Could you check a few things on this model? Use its own coordinates, in mm. A direction names the side the tool comes from. Round coordinates to 2 decimals unless told otherwise and drop trailing zeros. Loops run counter-clockwise (first coordinate to the right, second up) from the corner with the lowest first, then second, coordinate; pieces in that order, holes last. Notation, with made-up numbers: (29.5, 65) -> (41.5, 65) arc R16 cw to (41.5, 69) -> close; hole circle Ø3 at (-5.75, 33). An arc over 180 degrees is marked (long way). Put each result on its own line as item: value. Start each with the question number.
1. Which directions (+Z, -Z, +X, -X, +Y, -Y) give clear straight access to the entire face, cutting with the end or side of a thin tool? Please do faces 4 (the flat face through (29.75, 2, 19)), 5 (the cylindrical face through (22.57, 1.77, 37.4)).
2. I'm going to push a flat-ended pin straight in: P1, Ø3, axis at x = 34, z = 34, coming from the +Y side. Where does the tip first touch, or does it pass through?
3. Imagine slicing it at D-D, the plane x = 25.5. Please give me the cut outline in (y, z), and give its area (3 significant figures).
4. Imagine slicing it at A-A, the plane z = 34. Count the separate pieces of the cut face and the enclosed holes in it, and give its area (3 significant figures).
5. Imagine slicing it at B-B, the plane x = 47. Please give me the cut outline in (y, z).
6. I need wall thicknesses on line 1 (Z direction, x = 34, y = 2.75); line 2 (X direction, y = 3.4, z = 27); line 3 (Z direction, x = 26, y = 1.1). Which ranges of each line are inside material? Lowest first, please. Write a range as [from, to].
7. If we mould it in two halves opening along Z, with no side actions, what happens to faces 1 (the cylindrical face through (75.86, 1.83, 33.41)), 2 (the cylindrical face through (77.4, 1.77, 37.43)), 3 (the flat face through (22, 2, 19))? For each: pulls with the +Z half, pulls with the -Z half, needs draft (parallel to the pull), parting line crosses it, or undercut.
8. Imagine slicing it at C-C, the plane z = 14. Please give me the cut outline in (x, y).
```python
from build123d import *

# Parameters (mm, degrees)
BOSS_EXTRUDE1_DEPTH = 3.6
SKETCH2_R           = 1.95
SKETCH2_W           = 39.75
SKETCH2_H           = 20
CUT_EXTRUDE1_DEPTH  = 3.6
SKETCH4_W           = 22
SKETCH4_H           = 38
CUT_EXTRUDE2_DEPTH  = 10
FILLET1_R           = 2
FILLET2_R           = 2
FILLET3_R           = 2
FILLET4_R           = 2
SKETCH5_R           = 2.25
CUT_EXTRUDE3_DEPTH  = 10


with BuildPart() as part:
    # Sketch1 → Boss-Extrude1 (new body)
    with BuildSketch(Plane(origin=(0, 0, 0), x_dir=(1, 0, 0), z_dir=(0, 1, 0))):
        with BuildLine():
            Line((2, 0), (98, 0))
            ThreePointArc((98, 0), (99.414213562, -0.585786438), (100, -2))
            Line((100, -2), (100, -36))
            ThreePointArc((100, -36), (99.414213562, -37.414213562), (98, -38))
            Line((98, -38), (2, -38))
            ThreePointArc((2, -38), (0.585786438, -37.414213562), (0, -36))
            Line((0, -36), (0, -2))
            ThreePointArc((0, -2), (0.585786438, -0.585786438), (2, 0))
        make_face()
    extrude(amount=BOSS_EXTRUDE1_DEPTH)

    # Sketch2 → Cut-Extrude1 (cut)
    with BuildSketch(Plane(origin=(0, 3.6, 0), x_dir=(1, 0, 0), z_dir=(0, 1, 0))):
        with Locations((90, -4.00475022)):
            Circle(SKETCH2_R)
        with Locations((82, -4.00475022)):
            Circle(SKETCH2_R)
        with Locations((18, -4.00475022)):
            Circle(SKETCH2_R)
        with Locations((26, -4.00475022)):
            Circle(SKETCH2_R)
        with Locations((34, -4.00475022)):
            Circle(SKETCH2_R)
        with Locations((42, -4.00475022)):
            Circle(SKETCH2_R)
        with Locations((50, -4.00475022)):
            Circle(SKETCH2_R)
        with Locations((58, -4.00475022)):
            Circle(SKETCH2_R)
        with Locations((66, -4.00475022)):
            Circle(SKETCH2_R)
        with Locations((74, -4.00475022)):
            Circle(SKETCH2_R)
        with Locations((90, -34)):
            Circle(SKETCH2_R)
        with Locations((82, -34)):
            Circle(SKETCH2_R)
        with Locations((18, -34)):
            Circle(SKETCH2_R)
        with Locations((26, -34)):
            Circle(SKETCH2_R)
        with Locations((34, -34)):
            Circle(SKETCH2_R)
        with Locations((42, -34)):
            Circle(SKETCH2_R)
        with Locations((50, -34)):
            Circle(SKETCH2_R)
        with Locations((58, -34)):
            Circle(SKETCH2_R)
        with Locations((66, -34)):
            Circle(SKETCH2_R)
        with Locations((74, -34)):
            Circle(SKETCH2_R)
        with Locations((49.625, -19)):
            Rectangle(SKETCH2_W, SKETCH2_H)
    extrude(amount=-CUT_EXTRUDE1_DEPTH, mode=Mode.SUBTRACT)

    # Sketch4 → Cut-Extrude2 (cut)
    with BuildSketch(Plane(origin=(0, 3.6, 0), x_dir=(1, 0, 0), z_dir=(0, 1, 0))):
        with Locations((89, -19)):
            Rectangle(SKETCH4_W, SKETCH4_H)
        with Locations((11, -19)):
            Rectangle(SKETCH4_W, SKETCH4_H)
    extrude(amount=-CUT_EXTRUDE2_DEPTH, mode=Mode.SUBTRACT)

    # Fillet1
    fillet1_edges = [part.edges().sort_by_distance(p)[0] for p in [
        (22, 1.8, 0),
    ]]
    fillet(fillet1_edges, radius=FILLET1_R)

    # Fillet2
    fillet2_edges = [part.edges().sort_by_distance(p)[0] for p in [
        (22, 1.8, 38),
    ]]
    fillet(fillet2_edges, radius=FILLET2_R)

    # Fillet3
    fillet3_edges = [part.edges().sort_by_distance(p)[0] for p in [
        (78, 1.8, 38),
    ]]
    fillet(fillet3_edges, radius=FILLET3_R)

    # Fillet4
    fillet4_edges = [part.edges().sort_by_distance(p)[0] for p in [
        (78, 1.8, 0),
    ]]
    fillet(fillet4_edges, radius=FILLET4_R)

    # Sketch5 → Cut-Extrude3 (cut)
    with BuildSketch(Plane(origin=(0, 3.6, 0), x_dir=(1, 0, 0), z_dir=(0, 1, 0))):
        with Locations((73.75, -14)):
            Circle(SKETCH5_R)
        with Locations((73.75, -24)):
            Circle(SKETCH5_R)
        with Locations((25.5, -14)):
            Circle(SKETCH5_R)
        with Locations((25.5, -24)):
            Circle(SKETCH5_R)
    extrude(amount=-CUT_EXTRUDE3_DEPTH, mode=Mode.SUBTRACT)


solid = part.part
```
Entries:
1. face 4: +Y, -Y
1. face 5: +Z, -X, +Y, -Y
2. P1: through
3. outline: (0, 0) -> (3.6, 0) -> (3.6, 2.12) -> (0, 2.12) -> close; (0, 5.89) -> (3.6, 5.89) -> (3.6, 11.75) -> (0, 11.75) -> close; (0, 16.25) -> (3.6, 16.25) -> (3.6, 21.75) -> (0, 21.75) -> close; (0, 26.25) -> (3.6, 26.25) -> (3.6, 32.12) -> (0, 32.12) -> close; (0, 35.88) -> (3.6, 35.88) -> (3.6, 38) -> (0, 38) -> close
3. area: 77.3 mm^2
4. separate pieces: 8
4. enclosed holes: 0
4. area: 103 mm^2
5. outline: (0, 0) -> (3.6, 0) -> (3.6, 9) -> (0, 9) -> close; (0, 29) -> (3.6, 29) -> (3.6, 38) -> (0, 38) -> close
6. line 1: [0, 2.05], [5.95, 9], [29, 32.05], [35.95, 38]
6. line 2: [22, 29.75], [69.5, 78]
6. line 3: [0, 2.05], [5.95, 11.81], [16.19, 21.81], [26.19, 32.05], [35.95, 38]
7. face 1: undercut
7. face 2: pulls with the +Z half
7. face 3: needs draft
8. outline: (22, 0) -> (23.25, 0) -> (23.25, 3.6) -> (22, 3.6) -> close; (27.75, 0) -> (29.75, 0) -> (29.75, 3.6) -> (27.75, 3.6) -> close; (69.5, 0) -> (71.5, 0) -> (71.5, 3.6) -> (69.5, 3.6) -> close; (76, 0) -> (78, 0) -> (78, 3.6) -> (76, 3.6) -> close
